The model under review builds one solid part; all positions refer to its coordinate system, in mm. Face numbers are marked on the shaded views. A direction names the side the tool comes from. Coordinates: 2 decimals unless noted, no trailing zeros. Write each loop counter-clockwise with the first axis right and the second up, starting at its lowest first coordinate (ties: lowest second). Pieces come first, ordered by that corner, then holes. Notation, with made-up numbers: (11, 17.25) - (42, 17.25) arc R28 cw to (42, 52.25) - close; hole circle Ø9 at (31.25, 85.25). An arc over 180 degrees is marked (long way). Answer as CSV lines item,"result". Start each with the question number.
Autodesk Inventor part; units mm, degrees
ref_plane "YZ Plane" through (0, 0, 0) normal (1, 0, 0) x (0, 1, 0)
ref_plane "XZ Plane" through (0, 0, 0) normal (0, 1, 0) x (-1, 0, 0)
ref_plane "XY Plane" through (0, 0, 0) normal (0, 0, 1) x (1, 0, 0)
sketch "Sketch1" plane through (0, 0, 0) normal (0, 1, 0) x (-1, 0, 0)
  line L0 (0, 0) -> (10, 0)
  line L1 (10, 0) -> (10, -10)
  line L2 (10, -10) -> (0, -10)
  line L3 (0, -10) -> (0, 0)
  dimension "d0" = 10
  dimension "d1" = 10
extrude "Extrusion1" add sketch "Sketch1" along normal blind 10
sketch "Sketch2" plane through (0, 0, 0) normal (1, 0, 0) x (0, 0, -1)
  line L0 (0, 10) -> (10, 10)
  line L1 (0, 0) -> (0, 10)
  line L2 (0, 5) -> (5, 10)
  line L3 (0, 10) -> (0, 5)
extrude "Extrusion2" cut sketch "Sketch2" against normal blind 10
sketch "Sketch3" plane through (0, 0, 0) normal (1, 0, 0) x (0, 0, -1)
  line L0 (10, 0) -> (10, 10)
  line L1 (5, 10) -> (10, 10)
  line L2 (8, 10) -> (8, 5)
  line L3 (8, 5) -> (10, 0)
  line L4 (10, 10) -> (8, 10)
extrude "Extrusion3" cut sketch "Sketch3" against normal blind 10
properties part number "141"
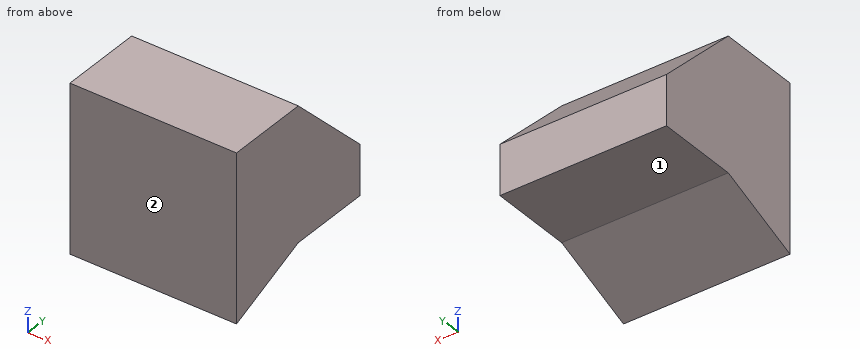
(1) Wall thickness on line 1 (Z direction, x = -6, y = 7.25); line 2 (Y direction, x = -7.5, z = -0.5); line 3 (Y direction, x = -2.25, z = -4.75): over which ranges is each line inside the solid? List them lowest first.
(2) For pin 1 (4 mm diameter, centred on x = -1, z = -2.5, fed in from +Y); pin 2 (3 mm diameter, centred on x = -4, y = 2, fed in from -Z); pin 3 (1.5 mm diameter, centred on x = -5, y = 8, fed in from -Z), all flat-tipped, find the tip position at first contact; note any pin that passes through.
(3) For the marked faces 1 and 2, list the 3-axis set-ups (+Z, -Z, +X, -X, +Y, -Y) from which the entire face can be reached by the end or side of a thin tool; tool diameter is ignored.
(4) Add section C-C on y = 1. Give the boundary of the cut face in (x, z), then the cut area to 3 significant figures.
(5) Add section A-A on x = -2.25. Give the boundary of the cut face in (y, z).
(6) Add section B-B on z = -3.5. Give the boundary of the cut face in (x, y), then the cut area to 3 significant figures.
Reported:
1,line 1,"-8 to -2.25"
1,line 2,"0 to 5.5"
1,line 3,"0 to 9.75"
2,pin 1,"y = 9.5"
2,pin 2,"z = -9.8"
2,pin 3,"z = -8"
3,face 1,"-Z, +X, -X, +Y"
3,face 2,"+Z, -Z, +X, -X, -Y"
4,outline,"(-10, -9.6) - (0, -9.6) - (0, 0) - (-10, 0) - close"
4,area,"96.0 mm²"
5,outline,"(0, -10) - (5, -8) - (10, -8) - (10, -5) - (5, 0) - (0, 0) - close"
6,outline,"(-10, 0) - (0, 0) - (0, 8.5) - (-10, 8.5) - close"
6,area,"85.0 mm²"
